```python
from build123d import *

# Parameters (mm, degrees)
SKETCH1_W           = 384.8
SKETCH1_H           = 497.2
BOSS_EXTRUDE1_DEPTH = 4
SKETCH2_W           = 384.8
SKETCH2_H           = 497.2
SKETCH2_W_2         = 368.8
SKETCH2_H_2         = 481.2
BOSS_EXTRUDE2_DEPTH = 24


with BuildPart() as part:
    # Sketch1 → Boss-Extrude1 (new, symmetric)
    with BuildSketch(Plane(origin=(0, 0, 0), x_dir=(1, 0, 0), z_dir=(0, 1, 0))):
        Rectangle(SKETCH1_W, SKETCH1_H)
    extrude(amount=BOSS_EXTRUDE1_DEPTH, both=True)

    # Sketch2 → Boss-Extrude2 (add)
    with BuildSketch(Plane(origin=(0, 4, 0), x_dir=(1, 0, 0), z_dir=(0, 1, 0))):
        Rectangle(SKETCH2_W, SKETCH2_H)
        Rectangle(SKETCH2_W_2, SKETCH2_H_2, mode=Mode.SUBTRACT)
    extrude(amount=BOSS_EXTRUDE2_DEPTH)


solid = part.part
```
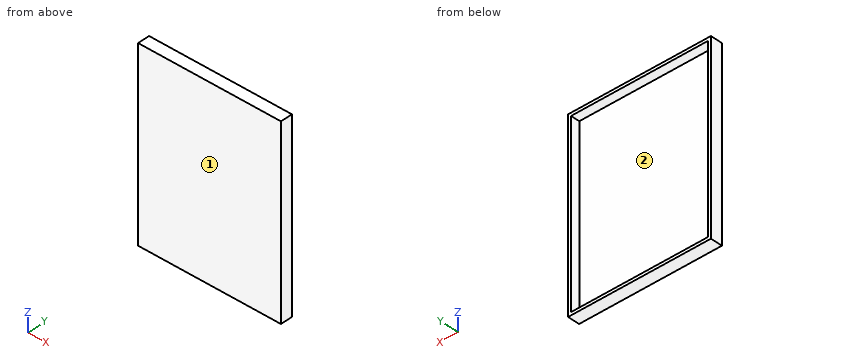
Input: part model. Units: mm. Frame: model coordinates. Face numbers are marked on the shaded views. Round coordinates to 2 decimals unless told otherwise and drop trailing zeros. Loops run counter-clockwise (first coordinate to the right, second up) from the corner with the lowest first, then second, coordinate; pieces in that order, holes last. Notation, with made-up numbers: (83.25, 52) - (113.25, 52) arc R28 cw to (113.25, 73) - close; hole circle Ø3 at (13.25, 16.25). An arc over 180 degrees is marked (long way). One line per item, written item: value. Start each with the question number.
(1) Draft query along Z for the marked faces 1 and 2. Return one class per face: +Z half, -Z half, draft (parallel to the pull), parting line (faces both ways), or undercut.
(2) Ray query, line 1 (X direction, y = 26.5, z = -93.5); line 2 (Z direction, x = 105, y = 7.5); line 3 (Y direction, x = -71.5, z = 202.5). Return the intervals inside material, ascending. Write a range as [from, to].
(3) Contact query for a flat-ended pin moving along its axis: P1, Ø5, axis at x = -49, z = -54, coming from the +Y side. Output: stop coordinate, or through.
(4) Section A-A, the plane y = 11. Return loops of the section in (x, z).
(5) Section C-C, the plane x = 35. Return loops of the section in (y, z).
(6) Section B-B, the plane z = 84. Return loops of the section in (x, y).
Results below:
1. face 1: draft
1. face 2: undercut
2. line 1: [-192.4, -184.4], [184.4, 192.4]
2. line 2: [-248.6, -240.6], [240.6, 248.6]
2. line 3: [-4, 4]
3. P1: y = 4
4. outline: (-192.4, -248.6) - (192.4, -248.6) - (192.4, 248.6) - (-192.4, 248.6) - close; hole (-184.4, -240.6) - (184.4, -240.6) - (184.4, 240.6) - (-184.4, 240.6) - close
5. outline: (-4, -248.6) - (28, -248.6) - (28, -240.6) - (4, -240.6) - (4, 240.6) - (28, 240.6) - (28, 248.6) - (-4, 248.6) - close
6. outline: (-192.4, -4) - (192.4, -4) - (192.4, 28) - (184.4, 28) - (184.4, 4) - (-184.4, 4) - (-184.4, 28) - (-192.4, 28) - close
